from build123d import *

# Parameters (mm, degrees)
BOSS_EXTRUDE1_DEPTH = 12
BOSS_EXTRUDE1_TAPER = 5
CUT_EXTRUDE1_DEPTH  = 10
CUT_EXTRUDE1_DRAFT  = -5
CUT_EXTRUDE2_DEPTH  = 1
FILLET1_R           = 2


with BuildPart() as part:
    # Sketch1 → Boss-Extrude1 (new body)
    with BuildSketch(Plane(origin=(0, 0, 0), x_dir=(1, 0, 0), z_dir=(0, 1, 0))):
        Polygon((71.807612477, 0), (35.903806238, 62.18721659), (-35.903806238, 62.18721659), (-71.807612477, 0), (-35.903806238, -62.18721659), (35.903806238, -62.18721659), align=None)
    extrude(amount=BOSS_EXTRUDE1_DEPTH, taper=BOSS_EXTRUDE1_TAPER)


with BuildPart() as cut_extrude1_tool:
    # Sketch2 → Cut-Extrude1 (with draft: the straight prism first)
    with BuildSketch(Plane.XZ):
        Polygon((68.704682034, 0), (34.352341017, 59.5), (-34.352341017, 59.5), (-68.704682034, 0), (-34.352341017, -59.5), (34.352341017, -59.5), align=None)
    extrude(amount=-CUT_EXTRUDE1_DEPTH)
    # Cut-Extrude1: the draft: its side faces are tilted about the plane it starts from
    cut_extrude1_sides = [cut_extrude1_tool.faces().sort_by_distance(p)[0] for p in [
        (51.528511525, 5, 29.75),
        (0, 5, 59.5),
        (-51.528511525, 5, 29.75),
        (-51.528511525, 5, -29.75),
        (0, 5, -59.5),
        (51.528511525, 5, -29.75),
    ]]
    draft(cut_extrude1_sides, Plane.XZ, CUT_EXTRUDE1_DRAFT)


with BuildPart() as part_1:
    add(part.part)

    # Cut-Extrude1: cut by cut_extrude1_tool
    add(cut_extrude1_tool.part, mode=Mode.SUBTRACT)

    # Sketch3 → Cut-Extrude2 (cut)
    with BuildSketch(Plane.XZ):
        Polygon((70.436732841, 0), (35.218366421, 61), (-35.218366421, 61), (-70.436732841, 0), (-35.218366421, -61), (35.218366421, -61), align=None)
    extrude(amount=-CUT_EXTRUDE2_DEPTH, mode=Mode.SUBTRACT)

    # Fillet1
    fillet1_edges = [part_1.edges().sort_by_distance(p)[0] for p in [
        (35.600736618, 6, 61.662284609),
        (-35.600736618, 6, 61.662284609),
        (-71.201473236, 6, 0),
        (-35.600736618, 6, -61.662284609),
        (35.600736618, 6, -61.662284609),
        (71.201473236, 6, 0),
        (0, 12, -61.137352628),
        (-52.946500496, 12, -30.568676314),
        (-52.946500496, 12, 30.568676314),
        (0, 12, 61.137352628),
        (52.946500496, 12, 30.568676314),
        (52.946500496, 12, -30.568676314),
    ]]
    fillet(fillet1_edges, radius=FILLET1_R)


solid = part_1.part
Input: part model. Units: mm. Frame: model coordinates. A direction names the side the tool comes from. Give positions to 0.01 mm unless a question says otherwise; leave off trailing zeros. Write each question's results on one line, items separated by ' | '.
Item 1: Access query for faces 1 (the flat face through (-53, 0, 32)), 2 (the flat face through (-52.58, 0.49, 30.93)). Directions: +Z, -Z, +X, -X, +Y, -Y. A direction counts if a zero-diameter tool reaches every point of the face in a straight line with its end or side. Return the directions, or none.
A:
face 1: +Z, -Z, +X, -X, -Y | face 2: -Y
Item 2: Material intervals for line 1 along Z through (x, y) = (61.5, 5); line 2 along Y through (x, z) = (-10, -34.5); line 3 along Z through (x, y) = (-21, 6.75), sorted ascending.
A:
line 1: z = -16.98 to -11.6, 11.6 to 16.98 | line 2: y = 10 to 12 | line 3: z = -61.6 to -58.91, 58.91 to 61.6
Item 3: Contact query for flat-ended pins moving along their axis: pin 1 Ø5 at (y, z) = (2, -37) entering from +X; pin 2 Ø4 at (x, y) = (18, 3) entering from +Z; pin 3 Ø5 at (y, z) = (2.5, 26.5) entering from +X. Output: stop coordinate, or through.
A:
pin 1: stops at x = 51.71 | pin 2: stops at z = 62.1 | pin 3: stops at x = 57.72
Item 4: Draft query along X for faces 3 (the flat face through (53.074, 0.493, 30.073)), 4 (the flat face through (-53.074, 0.493, -30.073)), 5 (the flat face through (1, 12, -1)). Return one class per face: released by +X, released by -X, zero draft, split by the parting line, or undercut.
A:
face 3: undercut | face 4: undercut | face 5: zero draft
